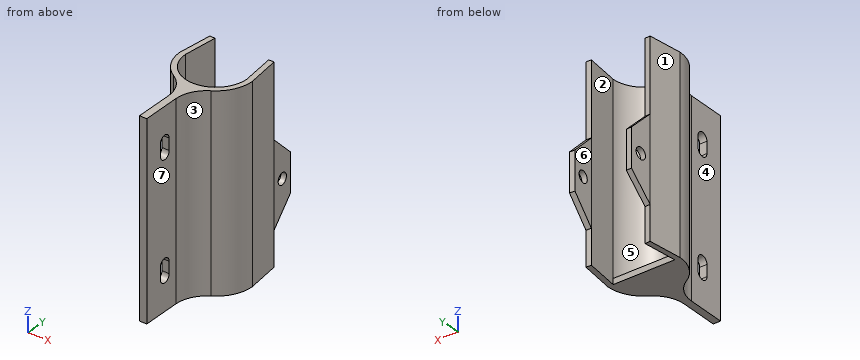
```python
from build123d import *

# Parameters (mm, degrees)
F1_DEPTH  = 1.5
F2_DEPTH  = 50
F3_R      = 8
F4_W      = 1.3695214008
F4_H      = 10
F6_DEPTH  = 6
F5_W      = 1.3695214008
F5_H      = 10
F7_DEPTH  = 6
F8_R      = 1.5
F9_DEPTH  = 2
F10_R     = 1.5
F11_DEPTH = 2
F12_SIZE  = 5.99999
F14_DEPTH = 3


# Not quite as in the source:
# - a fillet or chamfer is up to 0.001 mm smaller than in the source, because OpenCascade refuses the exact size


with BuildPart() as f1:
    # F0 (on Top) → F1 (new body)
    with BuildSketch(Plane.XY):
        with BuildLine():
            Line((-8.8714406544, -8.0876392549), (-13.1571549401, -8.0876392549))
            ThreePointArc((-13.1571549401, -8.0876392549), (-5.1571549401, -16.0876392549), (2.8428450599, -8.0876392549))
            Line((2.8428450599, -8.0876392549), (-1.4428692258, -8.0876392549))
            Line((-1.4428692258, -8.0876392549), (-8.8714406544, -8.0876392549))
        make_face()
    extrude(amount=F1_DEPTH)

    # F0 (on Top) → F2 (join)
    with BuildSketch(Plane.XY):
        with BuildLine():
            ThreePointArc((2.8428450599, -8.0876392549), (-5.1571549401, -16.0876392549), (-13.1571549401, -8.0876392549))
            Line((-13.1571549401, -8.0876392549), (-12.1455313702, 0.680061955))
            Line((-12.1455313702, 0.680061955), (-13.5133440803, 0.7484524309))
            Line((-13.5133440803, 0.7484524309), (-14.5857263686, -8.0876392549))
            ThreePointArc((-14.5857263686, -8.0876392549), (-12.1513540266, -14.4105450997), (-6.1053030882, -17.4684161029))
            Line((-6.1053030882, -17.4684161029), (-6.1053030882, -32.9236180908))
            Line((-6.1053030882, -32.9236180908), (-4.2090067919, -32.9236180908))
            Line((-4.2090067919, -32.9236180908), (-4.2090067919, -17.4684161029))
            ThreePointArc((-4.2090067919, -17.4684161029), (1.8370441464, -14.4105450997), (4.2714164885, -8.0876392549))
            Line((4.2714164885, -8.0876392549), (3.1990342002, 0.7484524309))
            Line((3.1990342002, 0.7484524309), (1.83122149, 0.680061955))
            Line((1.83122149, 0.680061955), (2.8428450599, -8.0876392549))
        make_face()
    extrude(amount=F2_DEPTH)

    # F3
    f3_edges = [f1.edges().sort_by_distance(p)[0] for p in [
        (-6.105303, -17.468416, 25),
        (-4.209007, -17.468416, 25),
    ]]
    fillet(f3_edges, radius=F3_R)

    # F4 (on face) → F6 (join)
    with BuildSketch(Plane(origin=(-0.0293516073, 0.5870335173, 0), x_dir=(-0.9987523447, -0.0499375007, 0), z_dir=(-0.0499375007, 0.9987523447, 0))):
        with Locations((-2.5476580515, 20)):
            Rectangle(F4_W, F4_H)
    extrude(amount=F6_DEPTH)

    # F5 (on face) → F7 (join)
    with BuildSketch(Plane(origin=(0.0036302561, 0.0726052918, 0), x_dir=(-0.9987523447, 0.0499375007, 0), z_dir=(0.0499375007, 0.9987523447, 0))):
        with Locations((12.8490992282, 20)):
            Rectangle(F5_W, F5_H)
    extrude(amount=F7_DEPTH)

    # F8 (on face) → F9 (cut)
    with BuildSketch(Plane(origin=(3.2283858075, 0.1614189135, 0), x_dir=(-0.0499375007, 0.9987523447, 0), z_dir=(0.9987523447, 0.0499375007, 0))):
        with Locations((3.5877668478, 20)):
            Circle(F8_R)
    extrude(amount=-F9_DEPTH, mode=Mode.SUBTRACT)

    # F10 (on face) → F11 (cut)
    with BuildSketch(Plane(origin=(-13.5169743364, 0.6758471391, 0), x_dir=(-0.0499375007, -0.9987523447, 0), z_dir=(-0.9987523447, 0.0499375007, 0))):
        with Locations((-3.0726959913, 20)):
            Circle(F10_R)
    extrude(amount=-F11_DEPTH, mode=Mode.SUBTRACT)

    # F12 (size 6 in the source; OpenCascade refuses exactly that, so slightly less here)
    f12_edges = [f1.edges().sort_by_distance(p)[0] for p in [
        (2.515128, 0.714257, 15),
        (-12.829438, 0.714257, 15),
        (2.515128, 0.714257, 25),
        (-12.829438, 0.714257, 25),
    ]]
    chamfer(f12_edges, length=F12_SIZE)

    # F13 (on face) → F14 (cut)
    with BuildSketch(Plane.YZ.offset(-4.2090067919)):
        with BuildLine():
            ThreePointArc((-28.2929875813, 38.5), (-26.7929875813, 37), (-25.2929875813, 38.5))
            Line((-25.2929875813, 38.5), (-25.2929875813, 41.5))
            ThreePointArc((-25.2929875813, 41.5), (-26.7929875813, 43), (-28.2929875813, 41.5))
            Line((-28.2929875813, 41.5), (-28.2929875813, 38.5))
        make_face()
        with BuildLine():
            ThreePointArc((-28.2929875813, 8.5), (-26.7929875813, 7), (-25.2929875813, 8.5))
            Line((-25.2929875813, 8.5), (-25.2929875813, 11.5))
            ThreePointArc((-25.2929875813, 11.5), (-26.7929875813, 13), (-28.2929875813, 11.5))
            Line((-28.2929875813, 11.5), (-28.2929875813, 8.5))
        make_face()
    extrude(amount=-F14_DEPTH, mode=Mode.SUBTRACT)


solid = f1.part
```
The model under review builds one solid part; all positions refer to its coordinate system, in mm. Face numbers are marked on the shaded views. A direction names the side the tool comes from. Round coordinates to 2 decimals unless told otherwise and drop trailing zeros. Loops run counter-clockwise (first coordinate to the right, second up) from the corner with the lowest first, then second, coordinate; pieces in that order, holes last.
1) Consider section D-D on y = -14.5. State the section outline as (x, z) points, then the cut area to 3 significant figures.
Values follow:
outline: (-12.07, 0) - (1.76, 0) - (1.76, 50) - (-0.37, 50) - (-0.37, 1.5) - (-9.94, 1.5) - (-9.94, 50) - (-12.07, 50) - close
area: 227 mm2
2) Consider section B-B on z = 46. State the section outline as (x, y) points.
Values follow:
outline: (-14.59, -8.09) arc R9.43 ccw to (-10, -16.18) arc R8 cw to (-6.11, -23.04) - (-6.11, -32.92) - (-4.21, -32.92) - (-4.21, -23.04) arc R8 cw to (-0.32, -16.18) arc R9.43 ccw to (4.27, -8.09) - (3.2, 0.75) - (1.83, 0.68) - (2.84, -8.09) arc R8 cw to (-13.16, -8.09) - (-12.15, 0.68) - (-13.51, 0.75) - close
3) Clearance check with flat-ended pins moving along their axes: P1, Ø8, axis at y = -28.5, z = 23.5, coming from the -X side; P2, Ø4, axis at x = -1.5, y = -12, coming from the +Z side; P3, Ø5, axis at y = -17.5, z = 9, coming from the +X side; P4, Ø8, axis at x = 1.5, y = -21, coming from the +Z side (3 decimals). State where each tip first meets the part, or that it passes through.
Values follow:
P1: stops at x = -6.11
P2: stops at z = 1.5
P3: stops at x = 1.26
P4: passes through
4) Tool access review of the marked faces 4, 5, 6 and 7: name each direction out of +Z, -Z, +X, -X, +Y, -Y from which nothing blocks a thin tool from reaching the whole face with its end or side.
Values follow:
face 4: +Z, -Z, -X, -Y
face 5: +Z
face 6: +Z, -Z
face 7: +Z, -Z, +X, -Y
5) Consider section C-C on x = -2. State the section outline as (y, z) points.
Values follow:
outline: (-17.52, 0) - (-8.09, 0) - (-8.09, 1.5) - (-15.44, 1.5) - (-15.44, 50) - (-17.52, 50) - close
6) Wall thickness on line 1 along X through (y, z) = (-24.5, 11); line 2 along X through (y, z) = (-13.5, 26.5); line 3 along X through (y, z) = (-12.5, 20): over which ranges is each line inside the solid? List them lowest first.
Values follow:
line 1: x = -6.11 to -4.21
line 2: x = -12.88 to -11.05, 0.73 to 2.56
line 3: x = -13.49 to -11.83, 1.52 to 3.18
7) Consider section A-A on y = -1.5. State the section outline as (x, z) points.
Values follow:
outline: (-13.79, 0) - (-12.4, 0) - (-12.4, 50) - (-13.79, 50) - close; (2.08, 0) - (3.47, 0) - (3.47, 50) - (2.08, 50) - close
8) The part is to be moulded in two halves that separate along Y. For the marked faces 1, 2 and 3, say which applies: pulls with the +Y half, pulls with the -Y half, needs draft (parallel to the pull), parting line crosses it, or undercut.
Values follow:
face 1: pulls with the +Y half
face 2: undercut
face 3: pulls with the -Y half
